Build history of the part. All positions in model axes, mm. Face numbers are marked on the shaded views. A direction names the side the tool comes from. Round coordinates to 2 decimals unless told otherwise and drop trailing zeros. Answer in a Markdown table with one row per item. Add a question column.
from build123d import *

# Parameters (mm, degrees)
F0_W     = 25.4
F0_H     = 25.4
F1_DEPTH = 12.7
F1_TAPER = -3
F2_T     = -2.54
F3_R     = 1.27


with BuildPart() as f1:
    # F0 (on Top) → F1 (new body)
    with BuildSketch(Plane.XY):
        Rectangle(F0_W, F0_H)
    extrude(amount=F1_DEPTH, taper=F1_TAPER)

    # F2
    f2_openings = [f1.faces().sort_by_distance(p)[0] for p in [
        (0, 0, 12.7),
    ]]
    offset(amount=F2_T, openings=f2_openings)

    # F3
    f3_edges = [f1.edges().sort_by_distance(p)[0] for p in [
        (0, -10.28963, 2.54),
        (-10.28963, 0, 2.54),
        (0, 10.28963, 2.54),
        (10.28963, 0, 2.54),
        (0, 10.822093, 12.7),
        (-10.822093, 0, 12.7),
        (0, -10.822093, 12.7),
        (10.822093, 0, 12.7),
        (-10.555862, -10.555862, 7.62),
        (10.555862, -10.555862, 7.62),
        (10.555862, 10.555862, 7.62),
        (-10.555862, 10.555862, 7.62),
    ]]
    fillet(f3_edges, radius=F3_R)


solid = f1.part
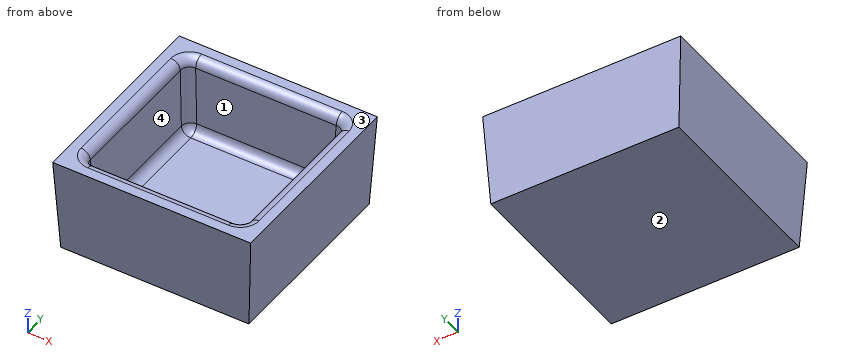
(1) Probe line 1 along X through (y, z) = (6.5, 9.75); line 2 along X through (y, z) = (-6, 6); line 3 along Y through (x, z) = (-3.5, 3.5). List the from-to ranges inside material, lowest first.
(2) Which spindle directions (+Z, -Z, +X, -X, +Y, -Y) get a long thin tool onto all of the face, cutting with end or side? Do the marked faces 1 and 2. Say none if no direction does.
(3) Drop flat-ended pins along their axis: P1, Ø5, axis at x = 4, y = -6.5, coming from the -Z side; P2, Ø2, axis at y = 4, z = 7, coming from the +X side; P3, Ø5, axis at y = -2.5, z = 6, coming from the -X side; P4, Ø3, axis at x = 8, y = -1, coming from the +Z side. Give the stop position or say it passes through.
(4) Mould opens along X. For the marked faces 3 and 4 say: pulls with the +X half, pulls with the -X half, needs draft (parallel to the pull), parting line crosses it, or undercut.
Answer sheet:
| question | item | result |
|---|---|---|
| 1 | line 1 | x = -13.21 to -10.67, 10.67 to 13.21 |
| 1 | line 2 | x = -13.01 to -10.47, 10.47 to 13.01 |
| 1 | line 3 | y = -12.88 to -10.32, 10.32 to 12.88 |
| 2 | face 1 | +Z |
| 2 | face 2 | -Z, +X, -X, +Y, -Y |
| 3 | P1 | stops at z = 0 |
| 3 | P2 | stops at x = 13.12 |
| 3 | P3 | stops at x = -13.15 |
| 3 | P4 | stops at z = 2.61 |
| 4 | face 3 | needs draft |
| 4 | face 4 | undercut |
